Geometry: final body of the model. Coordinates: model frame, mm. Give positions to 0.01 mm unless a question says otherwise; leave off trailing zeros. Loops run counter-clockwise (first coordinate to the right, second up) from the corner with the lowest first, then second, coordinate; pieces in that order, holes last.
from build123d import *

# Parameters (mm, degrees)
F0_W     = 50
F0_H     = 30
F0_R     = 3
F1_DEPTH = 10
F2_R     = 1


with BuildPart() as f1:
    # F0 (on Top) → F1 (new body)
    with BuildSketch(Plane.XY):
        with Locations((-25, 15)):
            Rectangle(F0_W, F0_H)
        with Locations((-38, 15)):
            Circle(F0_R, mode=Mode.SUBTRACT)
        with Locations((-12, 15)):
            Circle(F0_R, mode=Mode.SUBTRACT)
    extrude(amount=F1_DEPTH)

    # F2
    f2_edges = [f1.edges().sort_by_distance(p)[0] for p in [
        (-41, 15, 10),
        (-15, 15, 10),
    ]]
    fillet(f2_edges, radius=F2_R)


solid = f1.part
Item 1: Ray query, probe 1 along Y at (x, z) = (-38, 5); probe 2 along Y at (x, z) = (-14.5, 0.5); probe 3 along X at (y, z) = (13.5, 5.75). Return the intervals inside material, ascending.
Values follow:
probe 1: y = 0 to 12, 18 to 30
probe 2: y = 0 to 13.34, 16.66 to 30
probe 3: x = -50 to -40.6, -35.4 to -14.6, -9.4 to 0
Item 2: Section query A-A on y = 15. Return loops of the section in (x, z).
Values follow:
outline: (-50, 0) - (-41, 0) - (-41, 9) arc R1 ccw to (-42, 10) - (-50, 10) - close; (-35, 0) - (-15, 0) - (-15, 9) arc R1 ccw to (-16, 10) - (-34, 10) arc R1 ccw to (-35, 9) - close; (-9, 0) - (0, 0) - (0, 10) - (-8, 10) arc R1 ccw to (-9, 9) - close
Item 3: Section query B-B on x = -38. Return loops of the section in (y, z), plus the area to 3 significant figures.
Values follow:
outline: (0, 0) - (12, 0) - (12, 9) arc R1 ccw to (11, 10) - (0, 10) - close; (18, 0) - (30, 0) - (30, 10) - (19, 10) arc R1 ccw to (18, 9) - close
area: 240 mm2
Item 4: Draft query along X for faces 1 (the face through (-41, 15, 4)), 2 (the face through (-50, 15, 5)), 3 (the face through (-25, 15, 0)). Return one class per face: +X half, -X half, draft (parallel to the pull), parting line (faces both ways), or undercut.
Values follow:
face 1: undercut
face 2: -X half
face 3: draft
Item 5: Section query C-C on z = 8.5. Return loops of the section in (x, y), plus the area to 3 significant figures.
Values follow:
outline: (-50, 0) - (0, 0) - (0, 30) - (-50, 30) - close; hole circle Ø6 at (-38, 15); hole circle Ø6 at (-12, 15)
area: 1,440 mm2
Item 6: Pin query (flat end, axial travel): pin 1 (1.5 mm diameter, centred on y = 7, z = 4.5, fed in from +X). Return the tip coordinate at first contact, or that it passes through.
Values follow:
pin 1: stops at x = 0
